Build history of the part. All positions in model axes, mm. Face numbers are marked on the shaded views. A direction names the side the tool comes from. Coordinates: 2 decimals unless noted, no trailing zeros. Order: outer loops, then holes, each group sorted by start corner. A loop starts at its lowest first (then second) coordinate and runs counter-clockwise, first axis right, second up. Notation, with made-up numbers: (70, -34.5) - (109, -34.5) arc R25 cw to (109, -7.5) - close; hole circle Ø11 at (30, 15.25). An arc over 180 degrees is marked (long way). Write each question's results on one line, items separated by ' | '.
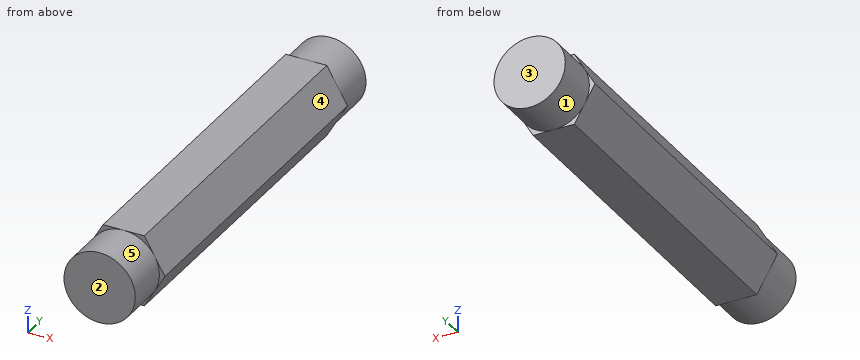
from build123d import *

# Parameters (mm, degrees)
BOSS_EXTRUDE1_DEPTH = 38.1
SKETCH2_OUTSIDE_W   = 32.39
SKETCH2_OUTSIDE_H   = 30.426
SKETCH2_OUTSIDE_R   = 6.35
CUT_EXTRUDE1_DEPTH  = 7.9502


with BuildPart() as part:
    # Sketch1 → Boss-Extrude1 (new, symmetric)
    with BuildSketch(Plane(origin=(0, 0, 0), x_dir=(1, 0, 0), z_dir=(0, 1, 0))):
        Polygon((3.666174209, -6.35), (7.332348419, 0), (3.666174209, 6.35), (-3.666174209, 6.35), (-7.332348419, 0), (-3.666174209, -6.35), align=None)
    extrude(amount=BOSS_EXTRUDE1_DEPTH, both=True)

    # Sketch2 outside → Cut-Extrude1 (cut)
    with BuildSketch(Plane(origin=(0, 38.1, 0), x_dir=(1, 0, 0), z_dir=(0, 1, 0))):
        Rectangle(SKETCH2_OUTSIDE_W, SKETCH2_OUTSIDE_H)
        with Locations(Location((0, 0, 0), (0, 0, 270))):
            Circle(SKETCH2_OUTSIDE_R, mode=Mode.SUBTRACT)
    cut_extrude1 = extrude(amount=-CUT_EXTRUDE1_DEPTH, mode=Mode.SUBTRACT)

    # Mirror1: Cut-Extrude1 across plane
    add(cut_extrude1.mirror(Plane.ZX), mode=Mode.SUBTRACT)


solid = part.part
1. Band-saw the part on B-B on x = 4.5. Give the cut face in (y, z), then the cut area to 3 significant figures.
Solved:
outline: (-38.1, -4.48) - (-30.15, -4.48) - (-30.15, -4.91) - (30.15, -4.91) - (30.15, -4.48) - (38.1, -4.48) - (38.1, 4.48) - (30.15, 4.48) - (30.15, 4.91) - (-30.15, 4.91) - (-30.15, 4.48) - (-38.1, 4.48) - close | area: 734 mm2
2. Drop flat-ended pins along their axis: pin 1 Ø1 at (y, z) = (13.5, -3) entering from -X; pin 2 Ø1.5 at (x, y) = (4.5, 10.5) entering from -Z; pin 3 Ø2 at (y, z) = (5, 4.5) entering from -X. Give the stop position or say it passes through.
Solved:
pin 1: stops at x = -5.89 | pin 2: stops at z = -6.2 | pin 3: stops at x = -5.31
3. Two-plate mould, pull along Y, no slides. Class the marked faces 1, 2 and 3: +Y half, -Y half, draft (parallel to the pull), parting line (faces both ways), or undercut.
Solved:
face 1: draft | face 2: -Y half | face 3: +Y half
4. Band-saw the part on A-A on y = -20.5. Give the cut face in (x, z), then the cut area to 3 significant figures.
Solved:
outline: (-7.33, 0) - (-3.67, -6.35) - (3.67, -6.35) - (7.33, 0) - (3.67, 6.35) - (-3.67, 6.35) - close | area: 140 mm2
5. Probe line 1 (X direction, y = 15, z = -4.75); line 2 (X direction, y = -13.5, z = 3); line 3 (Z direction, x = 4.75, y = -23). List the from-to ranges inside material, lowest first.
Solved:
line 1: x = -4.59 to 4.59 | line 2: x = -5.6 to 5.6 | line 3: z = -4.47 to 4.47
6. Tool access for the marked faces 4 and 5: list every direction of +Z, -Z, +X, -X, +Y, -Y with a clear straight run to the whole face (end or side of a thin tool).
Solved:
face 4: +Z, +X, +Y, -Y | face 5: -Y
